Part model, mm, in its own coordinate system. A direction names the side the tool comes from. Round coordinates to 2 decimals unless told otherwise and drop trailing zeros. Loops run counter-clockwise (first coordinate to the right, second up) from the corner with the lowest first, then second, coordinate; pieces in that order, holes last.
1) Band-saw the part on D-D, the plane y = -85. Write the cut outline in (x, z).
2) Drop flat-ended pins along their axis: P1, Ø3, axis at x = 55, y = -121, coming from the -Z side; P2, Ø21.5, axis at y = -22, z = 3.5, coming from the -X side; P3, Ø8, axis at x = 4, z = -6, coming from the +Y side; P4, Ø1, axis at y = -71, z = -32.5, coming from the +X side. Give the stop position or say it passes through.
3) Band-saw the part on B-B, the plane x = 11.5. Write the cut outline in (y, z), then the cut area to 3 significant figures.
4) Probe line 1 (Z direction, x = 44, y = -89); line 2 (Z direction, x = 57.5, y = -61.5); line 3 (Y direction, x = 57.5, z = -33). List the from-to ranges inside material, lowest first.
5) Band-saw the part on C-C, the plane z = 10.5. Write the cut outline in (x, y).
6) Mould opens along Z. For faces 5 (the flat face through (31, -72, -22.5)), 6 (the flat face through (52, -74, -44.5)), 7 (the cylindrical face through (45.975, -74.696, -34.36)) say: +Z half, -Z half, draft (parallel to the pull), parting line (faces both ways), or undercut.
7) 3-axis set-ups, long thin cutter, end or side, ignore diameter. For faces 1 (the cylindrical face through (45.975, -74.696, 34.36)), 2 (the flat face through (0, -22, 0)), 3 (the flat face through (2, -22, 0)), 4 (the cylindrical face through (6.393, -112.878, 0.315)): which of +Z, -Z, +X, -X, +Y, -Y reach the whole face in a straight line?
8) Band-saw the part on A-A, the plane y = -37. Write the cut outline in (x, z), then the cut area to 3 significant figures.
from build123d import *

# Parameters (mm, degrees)
BOSS_EXTRUDE1_DEPTH = 24.5
SHELL1_T            = -2
BOSS_EXTRUDE2_DEPTH = 20


with BuildPart() as part:
    # Sketch1 → Boss-Extrude1 (new body, symmetric)
    with BuildSketch(Plane.XY):
        with BuildLine():
            Line((0, 0), (65.97, 0))
            Line((65.97, 0), (65.97, -61.756344956))
            ThreePointArc((65.97, -61.756344956), (53.47, -74.256344956), (65.97, -86.756344956))
            Line((65.97, -86.756344956), (65.97, -147.256344956))
            ThreePointArc((65.97, -147.256344956), (4.282427581, -113.290220104), (0, -43))
            Line((0, -43), (0, 0))
        make_face()
    extrude(amount=BOSS_EXTRUDE1_DEPTH, both=True)

    # Shell1
    shell1_openings = [part.faces().sort_by_distance(p)[0] for p in [
        (32.985, 0, 0),
        (65.97, -30.878172478, 0),
        (59.72, -74.256344956, 0),
        (65.97, -117.006344956, 0),
    ]]
    offset(amount=SHELL1_T, openings=shell1_openings, kind=Kind.INTERSECTION)

    # Sketch2 → Boss-Extrude2 (add)
    with BuildSketch(Plane.XY.offset(24.5)):
        with BuildLine():
            Line((65.97, -54.256344956), (65.97, -61.756344956))
            ThreePointArc((65.97, -61.756344956), (53.47, -74.256344956), (65.97, -86.756344956))
            Line((65.97, -86.756344956), (65.97, -94.256344956))
            ThreePointArc((65.97, -94.256344956), (45.97, -74.256344956), (65.97, -54.256344956))
        make_face()
    boss_extrude2 = extrude(amount=BOSS_EXTRUDE2_DEPTH)

    # Mirror1: Boss-Extrude2 across plane
    add(boss_extrude2.mirror(Plane.XY))


solid = part.part
Reported:
1. outline: (-6.24, -24.5) - (49.1, -24.5) - (49.1, -44.5) - (59.58, -44.5) - (59.58, -22.5) - (-4.21, -22.5) - (-4.21, 22.5) - (59.58, 22.5) - (59.58, 44.5) - (49.1, 44.5) - (49.1, 24.5) - (-6.24, 24.5) - close
2. P1: stops at z = -24.5
2. P2: stops at x = 0
2. P3: stops at y = 0
2. P4: stops at x = 54.05
3. outline: (-122.86, -24.5) - (0, -24.5) - (0, -22.5) - (-119.8, -22.5) - (-119.8, 22.5) - (0, 22.5) - (0, 24.5) - (-122.86, 24.5) - close
3. area: 629 mm2
4. line 1: z = -24.5 to -22.5, 22.5 to 24.5
4. line 2: z = -44.5 to -22.5, 22.5 to 44.5
4. line 3: y = -92.37 to -83.45, -65.06 to -56.14
5. outline: (0, -43) arc R73 ccw to (65.97, -147.26) - (65.97, -145.26) arc R71 cw to (2, -43.45) - (2, 0) - (0, 0) - close
6. face 5: undercut
6. face 6: -Z half
6. face 7: draft
7. face 1: +Z, -X
7. face 2: +Z, -Z, -X, +Y
7. face 3: +X, +Y
7. face 4: +X
8. outline: (0, -24.5) - (65.97, -24.5) - (65.97, -22.5) - (2, -22.5) - (2, 22.5) - (65.97, 22.5) - (65.97, 24.5) - (0, 24.5) - close
8. area: 354 mm2
